Geometry: final body of the model. Coordinates: model frame, mm. Face numbers are marked on the shaded views. A direction names the side the tool comes from. Give positions to 0.01 mm unless a question says otherwise; leave off trailing zeros. Order: outer loops, then holes, each group sorted by start corner. A loop starts at its lowest first (then second) coordinate and runs counter-clockwise, first axis right, second up. Notation, with made-up numbers: (78.25, 52.25) - (96.25, 52.25) arc R25 ccw to (96.25, 83.25) - close; hole circle Ø6 at (25.5, -27). An arc over 180 degrees is marked (long way). Put each result on its own line as item: value. Start each with the question number.
1. Section D-D on z = 3.75. Count the separate pieces of the cut face and the enclosed holes in it, plus the area to 3 significant figures.
2. First-contact query: P1, Ø1.5, axis at y = 12.5, z = 8, coming from the +X side; P2, Ø12, axis at x = -3.5, y = 16, coming from the -Z side; P3, Ø3.5, axis at x = -33.5, y = 17, coming from the -Z side; P4, Ø4, axis at x = -0.5, z = 8.5, coming from the -Y side. Flat tips, straight axial feed; report the tip coordinate or a pass-through.
3. Section B-B on y = 53. Return the cut outline in (x, z), plus the area to 3 significant figures.
4. Set-up query: the marked faces 1, 2 and 3. Return all of +Z, -Z, +X, -X, +Y, -Y with unobstructed straight access to the full face (end or side cutting, diameter ignored); none if empty.
5. Section C-C on x = 29. Return the cut outline in (y, z).
6. Ray query, line 1 along X through (y, z) = (51.5, 1.5); line 2 along Y through (x, z) = (-33.5, 3.15); line 3 along Y through (x, z) = (-12.5, 2). Return the intervals inside material, ascending. Write a range as from..to.
7. Section A-A on y = 21. Return the cut outline in (x, z), plus the area to 3 significant figures.
8. Mould query, pull axis X, two halves, no side actions, for the marked faces 4 and 5. Classes: pulls with the +X half, pulls with the -X half, needs draft (parallel to the pull), parting line crosses it, or undercut.
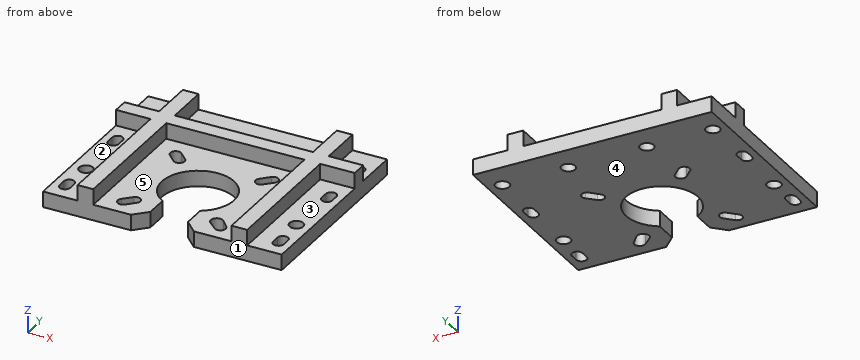
from build123d import *

# Parameters (mm, degrees)
SKETCH1_W           = 76
SKETCH1_H           = 62
BOSS_EXTRUDE1_DEPTH = 10
SKETCH2_W           = 44
SKETCH2_H           = 5
CUT_EXTRUDE1_DEPTH  = 43
CUT_EXTRUDE2_DEPTH  = 73.890328577
CUT_EXTRUDE3_DEPTH  = 73.890328577
CUT_EXTRUDE4_DEPTH  = 73.890328577
CUT_EXTRUDE5_DEPTH  = 73.890328577
CUT_EXTRUDE6_DEPTH  = 74.402997214
SKETCH8_W           = 11
SKETCH8_H           = 5
CUT_EXTRUDE7_DEPTH  = 43
CUT_EXTRUDE8_DEPTH  = 74.402997214
SKETCH10_W          = 11
SKETCH10_H          = 5
CUT_EXTRUDE9_DEPTH  = 43
CUT_EXTRUDE10_DEPTH = 73.890328577
CUT_EXTRUDE11_DEPTH = 74.402997214
CUT_EXTRUDE12_DEPTH = 73.890328577
SKETCH14_W          = 11
SKETCH14_H          = 5
CUT_EXTRUDE13_DEPTH = 14
SKETCH15_W          = 11
SKETCH15_H          = 5
CUT_EXTRUDE14_DEPTH = 14
SKETCH16_W          = 44
SKETCH16_H          = 5
CUT_EXTRUDE15_DEPTH = 14
SKETCH17_W          = 11.5
SKETCH17_H          = 5
HOLE1_D             = 4.4
HOLE2_D             = 4.4
HOLE3_D             = 4.4
HOLE4_D             = 4.4
HOLE5_D             = 4.4
HOLE6_D             = 4.4
CHAMFER1_SIZE       = 4
CHAMFER2_SIZE       = 4


with BuildPart() as part:
    # Sketch1 → Boss-Extrude1 (new body)
    with BuildSketch(Plane(origin=(0, 0, 0), x_dir=(-1, 0, 0), z_dir=(0, 0, -1))):
        with Locations((0, 31)):
            Rectangle(SKETCH1_W, SKETCH1_H)
    extrude(amount=-BOSS_EXTRUDE1_DEPTH)

    # Sketch2 → Cut-Extrude1 (cut)
    with BuildSketch(Plane.XZ):
        with Locations((0, 7.5)):
            Rectangle(SKETCH2_W, SKETCH2_H)
    extrude(amount=-CUT_EXTRUDE1_DEPTH, mode=Mode.SUBTRACT)

    # Sketch3 → Cut-Extrude2 (cut, through all)
    with BuildSketch(Plane.XY.offset(5)):
        with BuildLine():
            Line((-6, 0), (6, 0))
            Line((6, 0), (6, 11.192803568))
            ThreePointArc((6, 11.192803568), (0.00098815, 9.500001967), (-6, 11.185784174))
            Line((-6, 11.185784174), (-6, 0))
        make_face()
    extrude(amount=-CUT_EXTRUDE2_DEPTH, mode=Mode.SUBTRACT)

    # Sketch4 → Cut-Extrude3 (cut, through all)
    with BuildSketch(Plane.XY.offset(5)):
        with BuildLine():
            Line((-11.803657239, 35.202081528), (-14.303657239, 37.702081528))
            ThreePointArc((-14.303657239, 37.702081528), (-16.707820295, 37.702081528), (-16.707820295, 35.297918472))
            Line((-16.707820295, 35.297918472), (-14.207820295, 32.797918472))
            ThreePointArc((-14.207820295, 32.797918472), (-11.803657239, 32.797918472), (-11.803657239, 35.202081528))
        make_face()
    extrude(amount=-CUT_EXTRUDE3_DEPTH, mode=Mode.SUBTRACT)

    # Sketch5 → Cut-Extrude4 (cut, through all)
    with BuildSketch(Plane.XY.offset(5)):
        with BuildLine():
            Line((-14.207820295, 9.202081528), (-16.707820295, 6.702081528))
            ThreePointArc((-16.707820295, 6.702081528), (-16.707820295, 4.297918472), (-14.303657239, 4.297918472))
            Line((-14.303657239, 4.297918472), (-11.803657239, 6.797918472))
            ThreePointArc((-11.803657239, 6.797918472), (-11.803657239, 9.202081528), (-14.207820295, 9.202081528))
        make_face()
    extrude(amount=-CUT_EXTRUDE4_DEPTH, mode=Mode.SUBTRACT)

    # Sketch6 → Cut-Extrude5 (cut, through all)
    with BuildSketch(Plane.XY.offset(5)):
        with BuildLine():
            Line((11.730546448, 6.589437375), (14.359896375, 4.233818192))
            ThreePointArc((14.359896375, 4.233818192), (16.696342761, 4.297918472), (16.760443041, 6.634364857))
            Line((16.760443041, 6.634364857), (14.404823858, 9.263714785))
            ThreePointArc((14.404823858, 9.263714785), (11.655108147, 9.339153086), (11.730546448, 6.589437375))
        make_face()
    extrude(amount=-CUT_EXTRUDE5_DEPTH, mode=Mode.SUBTRACT)

    # Sketch7 → Cut-Extrude6 (cut, through all)
    with BuildSketch(Plane(origin=(0, 0, 0), x_dir=(-1, 0, 0), z_dir=(0, 0, -1))):
        with BuildLine():
            Line((-16.696342761, 35.297918472), (-14.196342761, 32.797918472))
            ThreePointArc((-14.196342761, 32.797918472), (-11.792179705, 32.797918472), (-11.792179705, 35.202081528))
            Line((-11.792179705, 35.202081528), (-14.292179705, 37.702081528))
            ThreePointArc((-14.292179705, 37.702081528), (-16.696342761, 37.702081528), (-16.696342761, 35.297918472))
        make_face()
    extrude(amount=-CUT_EXTRUDE6_DEPTH, mode=Mode.SUBTRACT)

    # Sketch8 → Cut-Extrude7 (cut)
    with BuildSketch(Plane.XZ):
        with Locations((32.5, 7.5)):
            Rectangle(SKETCH8_W, SKETCH8_H)
    extrude(amount=-CUT_EXTRUDE7_DEPTH, mode=Mode.SUBTRACT)

    # Sketch9 → Cut-Extrude8 (cut, through all)
    with BuildSketch(Plane(origin=(0, 0, 0), x_dir=(-1, 0, 0), z_dir=(0, 0, -1))):
        with BuildLine():
            Line((-32.3, 34), (-32.3, 36.5))
            ThreePointArc((-32.3, 36.5), (-34, 38.2), (-35.7, 36.5))
            Line((-35.7, 36.5), (-35.7, 34))
            ThreePointArc((-35.7, 34), (-34, 32.3), (-32.3, 34))
        make_face()
    extrude(amount=-CUT_EXTRUDE8_DEPTH, mode=Mode.SUBTRACT)

    # Sketch10 → Cut-Extrude9 (cut)
    with BuildSketch(Plane.XZ):
        with Locations((-32.5, 7.5)):
            Rectangle(SKETCH10_W, SKETCH10_H)
    extrude(amount=-CUT_EXTRUDE9_DEPTH, mode=Mode.SUBTRACT)

    # Sketch11 → Cut-Extrude10 (cut, through all)
    with BuildSketch(Plane.XY.offset(5)):
        with BuildLine():
            Line((-35.7, 36.5), (-35.7, 34))
            ThreePointArc((-35.7, 34), (-34, 32.3), (-32.3, 34))
            Line((-32.3, 34), (-32.3, 36.5))
            ThreePointArc((-32.3, 36.5), (-34, 38.2), (-35.7, 36.5))
        make_face()
    extrude(amount=-CUT_EXTRUDE10_DEPTH, mode=Mode.SUBTRACT)

    # Sketch12 → Cut-Extrude11 (cut, through all)
    with BuildSketch(Plane(origin=(0, 0, 0), x_dir=(-1, 0, 0), z_dir=(0, 0, -1))):
        with BuildLine():
            Line((32.3, 8), (32.3, 5.5))
            ThreePointArc((32.3, 5.5), (34, 3.8), (35.7, 5.5))
            Line((35.7, 5.5), (35.7, 8))
            ThreePointArc((35.7, 8), (34, 9.7), (32.3, 8))
        make_face()
    extrude(amount=-CUT_EXTRUDE11_DEPTH, mode=Mode.SUBTRACT)

    # Sketch13 → Cut-Extrude12 (cut, through all)
    with BuildSketch(Plane.XY.offset(5)):
        with BuildLine():
            Line((35.7, 5.5), (35.7, 8))
            ThreePointArc((35.7, 8), (34, 9.7), (32.3, 8))
            Line((32.3, 8), (32.3, 5.5))
            ThreePointArc((32.3, 5.5), (34, 3.8), (35.7, 5.5))
        make_face()
    extrude(amount=-CUT_EXTRUDE12_DEPTH, mode=Mode.SUBTRACT)

    # Sketch14 → Cut-Extrude13 (cut)
    with BuildSketch(Plane(origin=(0, 62, 0), x_dir=(-1, 0, 0), z_dir=(0, 1, 0))):
        with Locations((-32.5, 7.5)):
            Rectangle(SKETCH14_W, SKETCH14_H)
    extrude(amount=-CUT_EXTRUDE13_DEPTH, mode=Mode.SUBTRACT)

    # Sketch15 → Cut-Extrude14 (cut)
    with BuildSketch(Plane(origin=(0, 62, 0), x_dir=(-1, 0, 0), z_dir=(0, 1, 0))):
        with Locations((32.5, 7.5)):
            Rectangle(SKETCH15_W, SKETCH15_H)
    extrude(amount=-CUT_EXTRUDE14_DEPTH, mode=Mode.SUBTRACT)

    # Sketch16 → Cut-Extrude15 (cut)
    with BuildSketch(Plane(origin=(0, 62, 0), x_dir=(-1, 0, 0), z_dir=(0, 1, 0))):
        with Locations((0, 7.5)):
            Rectangle(SKETCH16_W, SKETCH16_H)
    extrude(amount=-CUT_EXTRUDE15_DEPTH, mode=Mode.SUBTRACT)

    # Sketch17 → Cut-Revolve1 (revolve, cut)
    with BuildSketch(Plane(origin=(0, 21, 0), x_dir=(-1, 0, 0), z_dir=(0, 1, 0))):
        with Locations((-5.744261233, 2.5)):
            Rectangle(SKETCH17_W, SKETCH17_H)
    revolve(axis=Axis((-0.005738767, 21, 0), (0, 0, 1)), mode=Mode.SUBTRACT)

    # Hole1 (through all)
    with Locations(Plane.XY.offset(5)):
        with Locations((-33.5, 17)):
            Hole(HOLE1_D / 2)

    # Hole2 (through all)
    with Locations(Plane.XY.offset(5)):
        with Locations((33.5, 17)):
            Hole(HOLE2_D / 2)

    # Hole3 (through all)
    with Locations(Plane.XY.offset(5)):
        with Locations((33.5, 53)):
            Hole(HOLE3_D / 2)

    # Hole4 (through all)
    with Locations(Plane.XY.offset(5)):
        with Locations((-33.5, 53)):
            Hole(HOLE4_D / 2)

    # Hole5 (through all)
    with Locations(Plane.XY.offset(5)):
        with Locations((-12.5, 53)):
            Hole(HOLE5_D / 2)

    # Hole6 (through all)
    with Locations(Plane.XY.offset(5)):
        with Locations((12.5, 53)):
            Hole(HOLE6_D / 2)

    # Chamfer1
    chamfer1_edges = [part.edges().sort_by_distance(p)[0] for p in [
        (-6, 0, 2.5),
    ]]
    chamfer(chamfer1_edges, length=CHAMFER1_SIZE)

    # Chamfer2
    chamfer2_edges = [part.edges().sort_by_distance(p)[0] for p in [
        (6, 0, 2.5),
    ]]
    chamfer(chamfer2_edges, length=CHAMFER2_SIZE)


solid = part.part
Resolved:
1. separate pieces: 1
1. enclosed holes: 14
1. area: 3,910 mm^2
2. P1: x = 27
2. P2: z = 0
2. P3: through
2. P4: y = 43
3. outline: (-38, 0) - (-35.7, 0) - (-35.7, 5) - (-38, 5) - close; (-31.3, 0) - (-14.7, 0) - (-14.7, 5) - (-22, 5) - (-22, 10) - (-27, 10) - (-27, 5) - (-31.3, 5) - close; (-10.3, 0) - (10.3, 0) - (10.3, 5) - (-10.3, 5) - close; (14.7, 0) - (31.3, 0) - (31.3, 5) - (27, 5) - (27, 10) - (22, 10) - (22, 5) - (14.7, 5) - close; (35.7, 0) - (38, 0) - (38, 5) - (35.7, 5) - close
3. area: 342 mm^2
4. face 1: +Z, -Z, +X, -X, -Y
4. face 2: +Z, -X, -Y
4. face 3: +Z, +X, -Y
5. outline: (0, 0) - (62, 0) - (62, 5) - (48, 5) - (48, 10) - (43, 10) - (43, 5) - (0, 5) - close
6. line 1: -38..-35.11, -31.89..-14.11, -10.89..10.89, 14.11..31.89, 35.11..38
6. line 2: 0..3.88, 9.62..14.8, 19.2..32.38, 38.12..50.8, 55.2..62
6. line 3: 0..6.1, 9.62..32.38, 35.9..50.8, 55.2..62
7. outline: (-38, 0) - (-11.51, 0) - (-11.51, 5) - (-22, 5) - (-22, 10) - (-27, 10) - (-27, 5) - (-38, 5) - close; (11.49, 0) - (38, 0) - (38, 5) - (27, 5) - (27, 10) - (22, 10) - (22, 5) - (11.49, 5) - close
7. area: 315 mm^2
8. face 4: needs draft
8. face 5: undercut
